Can you work these out from the drawing? Everything is in mm from the part's minimum corner. Give positions to 0.01 mm unless a question says otherwise; leave off trailing zeros. Write each loop counter-clockwise with the first axis right and the second up, starting at its lowest first coordinate (ties: lowest second). Pieces come first, ordered by that corner, then holes. Notation, with made-up numbers: M 61.25,84.25 L 72.25,84.25 A35 ccw 72.25,119.25 Z; hole C 27.25,71.25 d2. An arc over 180 degrees is marked long. One line per item, written item: value.
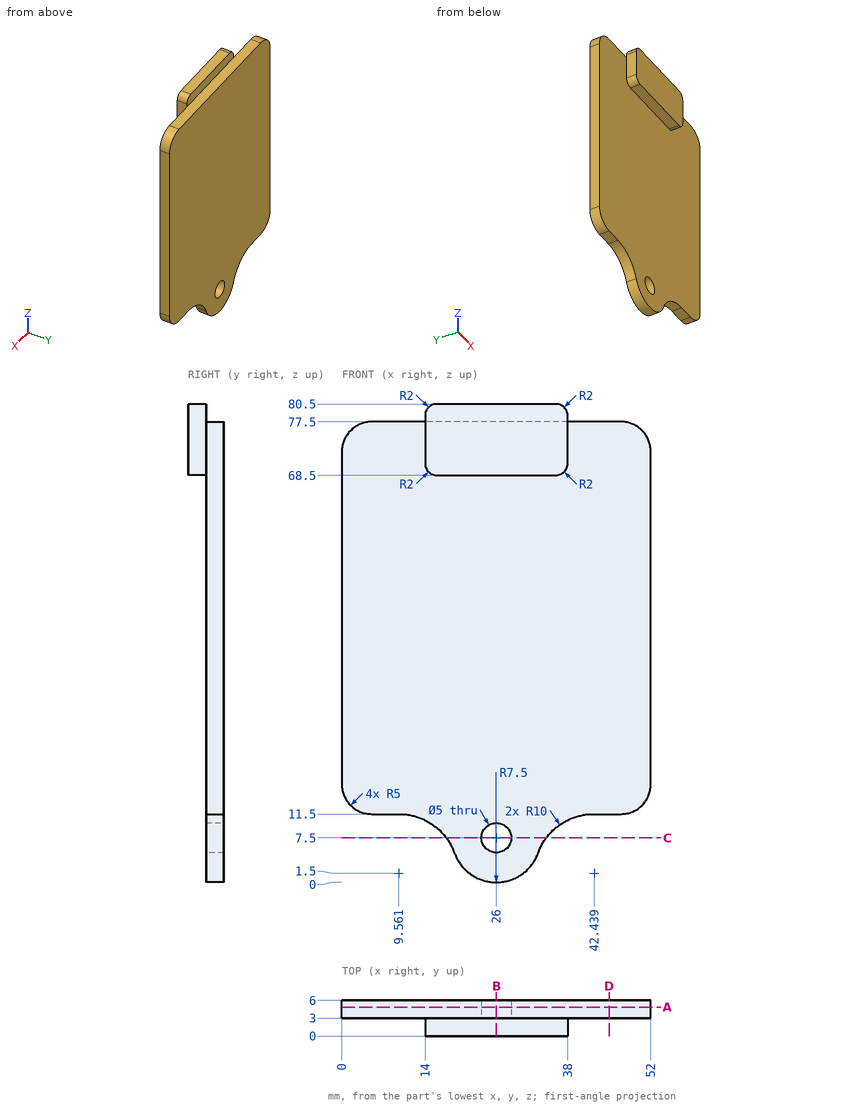
1) I'm going to push flat-ended pins straight in: pin 1 (5 mm diameter, centred on x = 27, z = 21.5, fed in from -Y); pin 2 (2.5 mm diameter, centred on x = 18.5, y = 4.5, fed in from +Z); pin 3 (0.9 mm diameter, centred on y = 1.5, z = 76, fed in from +X). Where does each tip first touch, or does it pass through?
Outcome:
pin 1: stops at y = 3
pin 2: stops at z = 77.5
pin 3: stops at x = 38
2) If we section it at B-B, the plane x = 26: Write out the boundary of the cut face in (y, z).
Outcome:
outline: M 0,68.5 L 3,68.5 L 3,10 L 6,10 L 6,77.5 L 3,77.5 L 3,80.5 L 0,80.5 Z; M 3,0 L 6,0 L 6,5 L 3,5 Z
3) If we section it at C-C, the plane z = 7.5: Write out the boundary of the cut face in (x, y).
Outcome:
outline: M 17.56,3 L 23.5,3 L 23.5,6 L 17.56,6 Z; M 28.5,3 L 34.44,3 L 34.44,6 L 28.5,6 Z
4) Please list where these lines run through material, in increasing order: L1, parallel to Y at x = 45.5, z = 69; L2, parallel to Z at x = 32.5, y = 2.05; L3, parallel to X at y = 4.95, z = 7.5. Write a range as from..to.
Outcome:
L1: y = 3..6
L2: z = 68.5..80.5
L3: x = 17.56..23.5, 28.5..34.44
5) If we section it at A-A, the plane y = 4.85: Write out the boundary of the cut face in (x, z) (1 decimal), then the cut area to 3 significant figures.
Outcome:
outline: M 0,16.5 A5 ccw 5,11.5 L 9.6,11.5 A10 cw 19,4.9 A7.5 ccw 33,4.9 A10 cw 42.4,11.5 L 47,11.5 A5 ccw 52,16.5 L 52,72.5 A5 ccw 47,77.5 L 5,77.5 A5 ccw 0,72.5 Z; hole C 26,7.5 d5
area: 3,570 mm^2
6) If we section it at D-D, the plane x = 45: Write out the boundary of the cut face in (y, z).
Outcome:
outline: M 3,11.5 L 6,11.5 L 6,77.5 L 3,77.5 Z
